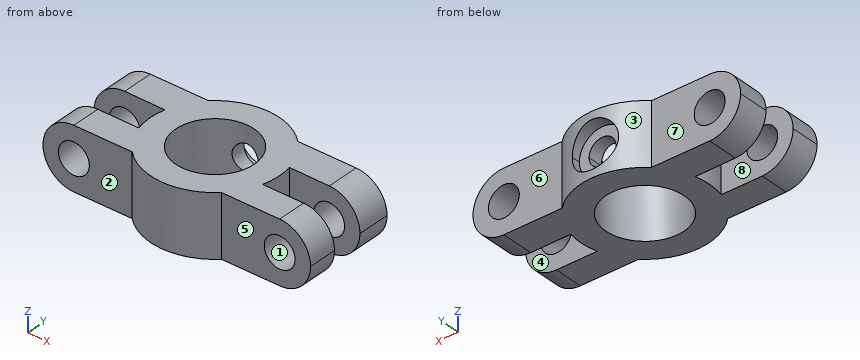
from build123d import *

# Parameters (mm, degrees)
F1_DEPTH  = 7.62
F3_DEPTH  = 7.62
F4_R      = 1.905
F5_DEPTH  = 11.431
F6_R      = 7.9375
F7_DEPTH  = 7.62
F8_R      = 4.826
F9_DEPTH  = 25.4
F11_DEPTH = 25.4
F14_DEPTH = 25.4


with BuildPart() as f1:
    # F0 (on Top) → F1 (new body)
    with BuildSketch(Plane.XY):
        Polygon((-16.51, -5.715), (0, -5.715), (16.51, -5.715), (16.51, 5.715), (-16.51, 5.715), align=None)
    extrude(amount=F1_DEPTH)

    # F2 (on face) → F3 (cut)
    with BuildSketch(Plane.XY.offset(7.62)):
        Polygon((-16.51, 1.905), (-16.51, 0), (-16.51, -2.138732), (16.51, -2.138732), (16.51, 1.671268), align=None)
    extrude(amount=-F3_DEPTH, mode=Mode.SUBTRACT)

    # F4 (on face) → F5 (cut, through all)
    with BuildSketch(Plane(origin=(0, 5.715, 0), x_dir=(-1, 0, 0), z_dir=(0, 1, 0))):
        with Locations((12.7, 3.81)):
            Circle(F4_R)
        with BuildLine():
            Line((16.51, 0), (16.51, 3.81))
            ThreePointArc((16.51, 3.81), (15.394077, 1.115923), (12.7, 0))
            Line((12.7, 0), (16.51, 0))
        make_face()
        with BuildLine():
            ThreePointArc((12.7, 7.62), (15.394077, 6.504077), (16.51, 3.81))
            Line((16.51, 3.81), (16.51, 7.62))
            Line((16.51, 7.62), (12.7, 7.62))
        make_face()
        with BuildLine():
            ThreePointArc((-10.795, 3.81), (-12.7, 5.715), (-14.605, 3.81))
            ThreePointArc((-14.605, 3.81), (-12.7, 1.905), (-10.795, 3.81))
        make_face()
        with BuildLine():
            Line((-16.51, 7.62), (-16.51, 3.81))
            ThreePointArc((-16.51, 3.81), (-15.394077, 6.504077), (-12.7, 7.62))
            Line((-12.7, 7.62), (-16.51, 7.62))
        make_face()
        with BuildLine():
            ThreePointArc((-12.7, 0), (-15.394077, 1.115923), (-16.51, 3.81))
            Line((-16.51, 3.81), (-16.51, 0))
            Line((-16.51, 0), (-12.7, 0))
        make_face()
    extrude(amount=-F5_DEPTH, mode=Mode.SUBTRACT)

    # F6 (on Top) → F7 (join, through all)
    with BuildSketch(Plane.XY):
        Circle(F6_R)
    extrude(amount=F7_DEPTH)

    # F8 (on face) → F9 (cut)
    with BuildSketch(Plane.XY.offset(7.62)):
        Circle(F8_R)
    extrude(amount=-F9_DEPTH, mode=Mode.SUBTRACT)

    # F10 (on Front) → F11 (cut)
    with BuildSketch(Plane.XZ):
        with BuildLine():
            ThreePointArc((0, 2.159), (1.167433, 2.642567), (1.651, 3.81))
            ThreePointArc((1.651, 3.81), (-1.167433, 4.977433), (0, 2.159))
        make_face()
    extrude(amount=-F11_DEPTH, mode=Mode.SUBTRACT)

    # F13 (on offset) → F14 (cut)
    with BuildSketch(Plane.XZ.offset(-6.35)):
        with BuildLine():
            ThreePointArc((0, 0.9525), (2.020558, 1.789442), (2.8575, 3.81))
            ThreePointArc((2.8575, 3.81), (-2.020558, 5.830558), (0, 0.9525))
        make_face()
    extrude(amount=-F14_DEPTH, mode=Mode.SUBTRACT)


solid = f1.part
The model under review builds one solid part; all positions refer to its coordinate system, in mm. Face numbers are marked on the shaded views. A direction names the side the tool comes from. Coordinates: 2 decimals unless noted, no trailing zeros. Write each loop counter-clockwise with the first axis right and the second up, starting at its lowest first coordinate (ties: lowest second). Pieces come first, ordered by that corner, then holes. Notation, with made-up numbers: (53.5, 23.5) - (64.5, 23.5) arc R10 cw to (64.5, 38.5) - close; hole circle Ø9 at (-2, 33.5). An arc over 180 degrees is marked (long way). Answer as a JSON object with one key per item and string values. Group by question number.
1. Clearance check with flat-ended pins moving along their axes: pin 1 Ø3 at (x, z) = (0, 2.5) entering from +Y; pin 2 Ø4 at (x, z) = (-12.5, 4.5) entering from -Y (3 decimals); pin 3 Ø2.5 at (x, z) = (-12.5, 5.5) entering from +Y (3 decimals). State where each tip first meets the part, or that it passes through.
2. Add section D-D (x = 4.5). Give the boundary of the cut face in (y, z).
3. Machinability: for the marked faces 4, 5, 6, 7 and 8, which of the approach directions +Z, -Z, +X, -X, +Y, -Y give a long, thin tool a straight path to every point of the face, cutting with its end or side? Answer none if there is none.
4. Add section A-A (y = 0). Give the boundary of the cut face in (x, z).
5. Add section B-B (y = -4.5). Give the boundary of the cut face in (x, z) (3 decimals).
6. To check wall thickness, follow probe 1 along X at (y, z) = (5.6, 3.81) (3 decimals); probe 2 along X at (y, z) = (3.15, 3.81) (3 decimals); probe 3 along Y at (x, z) = (-8, 0.5) (3 decimals). State the ranges of each line that lie inside material, in increasing order.
7. Add section C-C (x = -11.5). Give the boundary of the cut face in (y, z) (3 decimals), plus the area to 3 significant figures.
8. Mouldability with a two-part tool opening along X and no side actions: class the marked faces 1, 2 and 3 as pulls with the +X half, pulls with the -X half, needs draft (parallel to the pull), parting line crosses it, or undercut.
Findings:
{
 "1": {"pin 1": "y = 6.35", "pin 2": "y = -5.715", "pin 3": "y = 5.715"},
 "2": {"outline": "(-6.54, 0) - (-1.74, 0) - (-1.74, 7.62) - (-6.54, 7.62) - close; (1.74, 0) - (6.54, 0) - (6.54, 7.62) - (1.74, 7.62) - close"},
 "3": {"face 4": "+Z, -Z, +X", "face 5": "+Z, -Z, +X, -Y", "face 6": "+Z, -Z, +X, +Y", "face 7": "+Z, -Z, -X, +Y", "face 8": "+Z, -Z, -X"},
 "4": {"outline": "(-7.94, 0) - (-4.83, 0) - (-4.83, 7.62) - (-7.94, 7.62) - close; (4.83, 0) - (7.94, 0) - (7.94, 7.62) - (4.83, 7.62) - close"},
 "5": {"outline": "(-16.51, 3.81) arc R3.81 ccw to (-12.7, 0) - (-1.744, 0) - (-1.744, 7.62) - (-12.7, 7.62) arc R3.81 ccw to start; (1.744, 0) - (12.7, 0) arc R3.81 ccw to (16.51, 3.81) arc R3.81 ccw to (12.7, 7.62) - (1.744, 7.62) - close; hole circle Ø3.81 at (-12.7, 3.81); hole circle Ø3.81 at (12.7, 3.81)"},
 "6": {"probe 1": "-16.51 to -14.605, -10.795 to -1.651, 1.651 to 10.795, 14.605 to 16.51", "probe 2": "-16.51 to -14.605, -10.795 to -3.656, 3.656 to 10.795, 14.605 to 16.51", "probe 3": "-5.715 to -2.139, 1.845 to 5.715"},
 "7": {"outline": "(-5.715, 0) - (-2.139, 0) - (-2.139, 2.33) - (-5.715, 2.33) - close; (-5.715, 5.29) - (-2.139, 5.29) - (-2.139, 7.62) - (-5.715, 7.62) - close; (1.87, 0) - (5.715, 0) - (5.715, 2.33) - (1.87, 2.33) - close; (1.87, 5.29) - (5.715, 5.29) - (5.715, 7.62) - (1.87, 7.62) - close", "area": "34.6 mm²"},
 "8": {"face 1": "undercut", "face 2": "needs draft", "face 3": "parting line crosses it"}
}
